from build123d import *

# Parameters (mm, degrees)
F0_R     = 12.1
F0_R_2   = 8.1
F1_DEPTH = 6.4
F0_R_3   = 3.05
F2_DEPTH = 3
F3_R     = 8.1
F3_R_2   = 7.1
F4_DEPTH = 0.4


with BuildPart() as f1:
    # F0 (on Front) → F1 (new body)
    with BuildSketch(Plane.XZ):
        Circle(F0_R)
        Circle(F0_R_2, mode=Mode.SUBTRACT)
    extrude(amount=F1_DEPTH)

    # F0 (on Front) → F2 (join)
    with BuildSketch(Plane.XZ):
        with BuildLine():
            Line((-2.799697, -14.1), (2.799697, -14.1))
            ThreePointArc((2.799697, -14.1), (4.26998, -13.87894), (5.610256, -13.235306))
            Line((5.610256, -13.235306), (18.910559, -4.195761))
            ThreePointArc((18.910559, -4.195761), (20.518868, -2.400028), (21.1, -0.060455))
            Line((21.1, -0.060455), (21.1, 0.060455))
            ThreePointArc((21.1, 0.060455), (20.518868, 2.400028), (18.910559, 4.195761))
            Line((18.910559, 4.195761), (5.610256, 13.235306))
            ThreePointArc((5.610256, 13.235306), (4.26998, 13.87894), (2.799697, 14.1))
            Line((2.799697, 14.1), (-2.799697, 14.1))
            ThreePointArc((-2.799697, 14.1), (-4.26998, 13.87894), (-5.610256, 13.235306))
            Line((-5.610256, 13.235306), (-18.910559, 4.195761))
            ThreePointArc((-18.910559, 4.195761), (-20.518868, 2.400028), (-21.1, 0.060455))
            Line((-21.1, 0.060455), (-21.1, -0.060455))
            ThreePointArc((-21.1, -0.060455), (-20.518868, -2.400028), (-18.910559, -4.195761))
            Line((-18.910559, -4.195761), (-5.610256, -13.235306))
            ThreePointArc((-5.610256, -13.235306), (-4.26998, -13.87894), (-2.799697, -14.1))
        make_face()
        with Locations((-16.1, 0)):
            Circle(F0_R_3, mode=Mode.SUBTRACT)
        Circle(F0_R, mode=Mode.SUBTRACT)
        with Locations((16.1, 0)):
            Circle(F0_R_3, mode=Mode.SUBTRACT)
    extrude(amount=F2_DEPTH)

    # F3 (on face) → F4 (join)
    with BuildSketch(Plane(origin=(0, 0, 0), x_dir=(-1, 0, 0), z_dir=(0, 1, 0))):
        Circle(F3_R)
        Circle(F3_R_2, mode=Mode.SUBTRACT)
    extrude(amount=-F4_DEPTH)


solid = f1.part
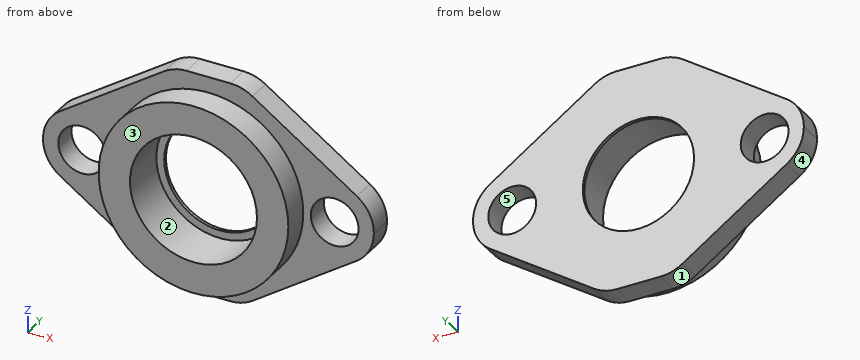
The model under review builds one solid part; all positions refer to its coordinate system, in mm. Face numbers are marked on the shaded views. A direction names the side the tool comes from. Round coordinates to 2 decimals unless told otherwise and drop trailing zeros. Loops run counter-clockwise (first coordinate to the right, second up) from the corner with the lowest first, then second, coordinate; pieces in that order, holes last. Notation, with made-up numbers: (81, 82) -> (126, 82) arc R16 cw to (126, 92) -> close; hole circle Ø2 at (-2.75, 29). An arc over 180 degrees is marked (long way). Write item = value, one per line. Start each with the question number.
Item 1: Take a section at C-C on x = 16.1. Give the boundary of the cut face in (y, z).
Item 2: Mouldability with a two-part tool opening along Z and no side actions: class the marked faces 3, 4 and 5 as released by +Z, released by -Z, zero draft, split by the parting line, or undercut.
Item 3: To check wall thickness, follow L1, parallel to Z at x = 0, y = -1.95; L2, parallel to Z at x = 0, y = -4.25; L3, parallel to Y at x = -12.5, z = 7. State the ranges of each line that lie inside material, in increasing order.
Item 4: Take a section at A-A on x = 0. Give the boundary of the cut face in (y, z), plus the area to 3 significant figures.
Item 5: Take a section at D-D on y = -5. Give the boundary of the cut face in (x, z).
Item 6: Insertion check: pin 1 (3 mm diameter, centred on y = -4, z = -11, fed in from -X); pin 2 (1 mm diameter, centred on x = -16.5, y = -1.5, fed in from -Z); pin 3 (2 mm diameter, centred on y = -5, z = 6.5, fed in from +X). Each pin has a flat end and moves straight along its axis. Give the tip position at first contact, or say it passes through.
Item 7: Take a section at B-B on y = -1.5. Give the boundary of the cut face in (x, z), plus the area to 3 significant figures.
Item 8: For the marked faces 1 and 2, list the 3-axis set-ups (+Z, -Z, +X, -X, +Y, -Y) from which the entire face can be reached by the end or side of a thin tool; tool diameter is ignored.
Result:
q1.outline = (-3, -6.11) -> (0, -6.11) -> (0, -3.05) -> (-3, -3.05) -> close; (-3, 3.05) -> (0, 3.05) -> (0, 6.11) -> (-3, 6.11) -> close
q2.face_3 = zero draft
q2.face_4 = released by -Z
q2.face_5 = undercut
q3.L1 = -14.1 to -8.1, 8.1 to 14.1
q3.L2 = -12.1 to -8.1, 8.1 to 12.1
q3.L3 = -3 to 0
q4.outline = (-6.4, -12.1) -> (-3, -12.1) -> (-3, -14.1) -> (0, -14.1) -> (0, -7.1) -> (-0.4, -7.1) -> (-0.4, -8.1) -> (-6.4, -8.1) -> close; (-6.4, 8.1) -> (-0.4, 8.1) -> (-0.4, 7.1) -> (0, 7.1) -> (0, 14.1) -> (-3, 14.1) -> (-3, 12.1) -> (-6.4, 12.1) -> close
q4.area = 64.0 mm²
q5.outline = circle Ø24.2 at (0, 0); hole circle Ø16.2 at (0, 0)
q6.pin_1 = -10.54
q6.pin_2 = -6.17
q6.pin_3 = 10.78
q7.outline = (-21.1, -0.06) arc R5 ccw to (-18.91, -4.2) -> (-5.61, -13.24) arc R5 ccw to (-2.8, -14.1) -> (2.8, -14.1) arc R5 ccw to (5.61, -13.24) -> (18.91, -4.2) arc R5 ccw to (21.1, -0.06) -> (21.1, 0.06) arc R5 ccw to (18.91, 4.2) -> (5.61, 13.24) arc R5 ccw to (2.8, 14.1) -> (-2.8, 14.1) arc R5 ccw to (-5.61, 13.24) -> (-18.91, 4.2) arc R5 ccw to (-21.1, 0.06) -> close; hole circle Ø6.1 at (-16.1, 0); hole circle Ø16.2 at (0, 0); hole circle Ø6.1 at (16.1, 0)
q7.area = 538 mm²
q8.face_1 = -Z, -X, +Y, -Y
q8.face_2 = -Y
